Check sheet for the modelled part. Datum: model origin and axes. Units: mm. Face numbers are marked on the shaded views. A direction names the side the tool comes from. Give positions to 0.01 mm unless a question says otherwise; leave off trailing zeros. Loops run counter-clockwise (first coordinate to the right, second up) from the corner with the lowest first, then second, coordinate; pieces in that order, holes last.
```python
from build123d import *

# Parameters (mm, degrees)
SKETCH_1_R          = 5
EXTRUDE_1_DEPTH     = 2
SKETCH_4_R          = 5.75
EXTRUDE_2_DEPTH     = 1
SKETCH_2_R          = 1.5
CUT_EXTRUDE_1_DEPTH = 5
SKETCH_3_R          = 4.1
SKETCH_3_R_2        = 2.54
CUT_EXTRUDE_2_DEPTH = 0.2


with BuildPart() as part:
    # 草圖1 → 填料-伸長1 (new body, symmetric)
    with BuildSketch(Plane.XY):
        Circle(SKETCH_1_R)
    extrude(amount=EXTRUDE_1_DEPTH, both=True)

    # 草圖4 → 填料-伸長2 (add)
    with BuildSketch(Plane(origin=(0, 0, -2), x_dir=(-1, 0, 0), z_dir=(0, 0, -1))):
        Circle(SKETCH_4_R)
    extrude(amount=-EXTRUDE_2_DEPTH)

    # 草圖2 → 除料-伸長1 (cut, through all)
    with BuildSketch(Plane.XY.offset(2)):
        Circle(SKETCH_2_R)
    extrude(amount=-CUT_EXTRUDE_1_DEPTH, mode=Mode.SUBTRACT)

    # 草圖3 → 除料-伸長2 (cut)
    with BuildSketch(Plane.XY.offset(2)):
        Circle(SKETCH_3_R)
        Circle(SKETCH_3_R_2, mode=Mode.SUBTRACT)
    cut_extrude_2 = extrude(amount=-CUT_EXTRUDE_2_DEPTH, mode=Mode.SUBTRACT)

    # 鏡射1: 除料-伸長2 across plane
    add(cut_extrude_2.mirror(Plane.XY), mode=Mode.SUBTRACT)


solid = part.part
```
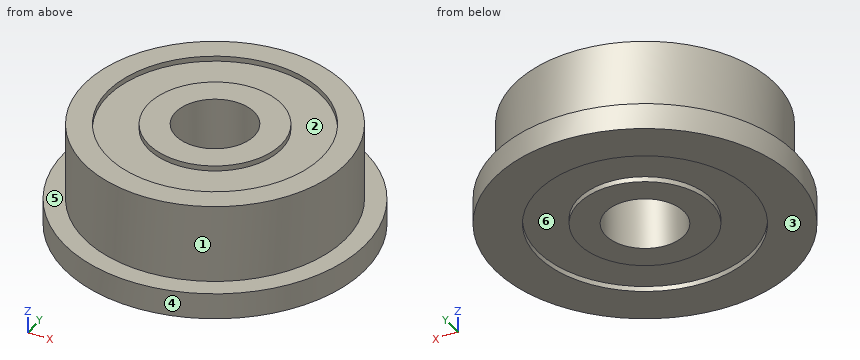
(1) Section check C-C on z = 1.45. Record the boundary of the cut face in (x, y).
(2) Gauge pin test, flat end, axial feed: pin 1 Ø5 at (x, y) = (0, 0) entering from +Z. Record the tip position at first contact, or that the pin passes through.
(3) Section check D-D on y = 4.5. Record the boundary of the cut face in (x, z).
(4) Release check for a two-part mould opening along Y. For the marked faces 1, 2 and 3 record: pulls with the +Y half, pulls with the -Y half, needs draft (parallel to the pull), parting line crosses it, or undercut.
(5) Access from +Z, -Z, +X, -X, +Y, -Y to the whole of each face (thin tool, end or side, straight path). Record for the marked faces 4, 5 and 6.
(6) Material ranges on line 1 (Y direction, x = 0, z = -1.9); line 2 (Z direction, x = -1.5, y = 2.75); line 3 (X direction, y = 1.25, z = -0.8), recorded low to high.
(7) Section check A-A on y = 0. Record the boundary of the cut face in (x, z).
Computed values:
1. outline: circle Ø10 at (0, 0); hole circle Ø3 at (0, 0)
2. pin 1: stops at z = 2
3. outline: (-3.58, -2) - (3.58, -2) - (3.58, -1) - (2.18, -1) - (2.18, 2) - (-2.18, 2) - (-2.18, -1) - (-3.58, -1) - close
4. face 1: parting line crosses it
4. face 2: undercut
4. face 3: needs draft
5. face 4: +Z, -Z
5. face 5: +Z
5. face 6: -Z
6. line 1: y = -5.75 to -4.1, -2.54 to -1.5, 1.5 to 2.54, 4.1 to 5.75
6. line 2: z = -1.8 to 1.8
6. line 3: x = -4.84 to -0.83, 0.83 to 4.84
7. outline: (-5.75, -2) - (-4.1, -2) - (-4.1, -1.8) - (-2.54, -1.8) - (-2.54, -2) - (-1.5, -2) - (-1.5, 2) - (-2.54, 2) - (-2.54, 1.8) - (-4.1, 1.8) - (-4.1, 2) - (-5, 2) - (-5, -1) - (-5.75, -1) - close; (1.5, -2) - (2.54, -2) - (2.54, -1.8) - (4.1, -1.8) - (4.1, -2) - (5.75, -2) - (5.75, -1) - (5, -1) - (5, 2) - (4.1, 2) - (4.1, 1.8) - (2.54, 1.8) - (2.54, 2) - (1.5, 2) - close
